Input: part model. Units: mm. Frame: model coordinates. A direction names the side the tool comes from. Give positions to 0.01 mm unless a question says otherwise; leave off trailing zeros. Write each loop counter-clockwise with the first axis right and the second up, starting at its lowest first coordinate (ties: lowest second). Pieces come first, ordered by that corner, then holes. Notation, with made-up numbers: (-36.5, 45.25) - (22.5, 45.25) arc R28 cw to (22.5, 84.25) - close; hole circle Ø1 at (24, -11.75). An arc over 180 degrees is marked (long way). Answer as a JSON object with one key per item and string values. Group by question number.
from build123d import *

# Parameters (mm, degrees)
F0_W     = 94
F0_H     = 148
F0_W_2   = 78
F0_H_2   = 136
F1_DEPTH = 2.5
F2_DEPTH = 3.2
F3_SIZE  = 3.19999
F6_DEPTH = 9
F7_R     = 5.99999
F8_R     = 2.5
F9_DEPTH = 12.1


# Not quite as in the source:
# - a fillet or chamfer is up to 0.001 mm smaller than in the source, because OpenCascade refuses the exact size


with BuildPart() as f1:
    # F0 (on Top) → F1 (new body)
    with BuildSketch(Plane.XY):
        Rectangle(F0_W, F0_H)
        with Locations((0, -2)):
            Rectangle(F0_W_2, F0_H_2, mode=Mode.SUBTRACT)
        with Locations((0, -2)):
            Rectangle(F0_W_2, F0_H_2)
    extrude(amount=-F1_DEPTH)

    # F0 (on Top) → F2 (join)
    with BuildSketch(Plane.XY):
        with Locations((0, -2)):
            Rectangle(F0_W_2, F0_H_2)
    extrude(amount=F2_DEPTH)

    # F3 (size 3.2 in the source; OpenCascade refuses exactly that, so slightly less here)
    f3_edges = [f1.edges().sort_by_distance(p)[0] for p in [
        (-39, -2, 3.2),
        (0, -70, 3.2),
        (39, -2, 3.2),
        (0, 66, 3.2),
    ]]
    chamfer(f3_edges, length=F3_SIZE)

    # F5 (on face) → F6 (join)
    with BuildSketch(Plane.XY.offset(3.2)):
        Polygon((-21.4385061716, 24.1024312943), (-19.825111455, 21.5732105668), (-14.9849273053, 13.9855483843), (-4.8680443952, 20.4391272506), (-11.3216232616, 30.5560101607), align=None)
    extrude(amount=F6_DEPTH)

    # F7 (radius 6 in the source; OpenCascade refuses exactly that, so slightly less here)
    f7_edges = [f1.edges().sort_by_distance(p)[0] for p in [
        (-9.926486, 17.212338, 12.2),
        (-16.380065, 27.329221, 12.2),
    ]]
    fillet(f7_edges, radius=F7_R)

    # F8 (on face) → F9 (cut)
    with BuildSketch(Plane(origin=(-4.3097861814, -2.749220809, 0), x_dir=(0.5377982389, -0.8430735758, 0), z_dir=(-0.8430735758, -0.5377982389, 0))):
        with Locations((-25.8497138006, 8.2)):
            Circle(F8_R)
    extrude(amount=-F9_DEPTH, mode=Mode.SUBTRACT)


solid = f1.part
1) Pin query (flat end, axial travel): P1, Ø4, axis at x = -17.5, y = 50.5, coming from the +Z side; P2, Ø6, axis at x = 16, z = 9, coming from the -Y side; P3, Ø1.5, axis at x = -28.5, z = 3, coming from the -Y side; P4, Ø4, axis at y = 27.5, z = 0.5, coming from the -X side. Return the tip coordinate at first contact, or that it passes through.
2) Cut plane C-C on z = 1.5. Return the cut outline in (x, y).
3) Line query: line 1 along Z through (x, y) = (19.5, 43.5); line 2 along Z through (x, y) = (40, 20.5); line 3 along Y through (x, z) = (-9.5, 7). Output: solid intervals per line, ascending. Write a range as from..to.
4) Reachability of faces 1 (the face through (-42, 6, 0)), 2 (the face through (-9.997, 17.167, 4.679)), 3 (the face through (-8.8, 26.6, 5.6)), 4 (the face through (-16.309, 27.374, 4.679)) from +Z, -Z, +X, -X, +Y, -Y: full face, straight path, thin tool, end or side. Return the list, or none.
5) Mould query, pull axis Z, two halves, no side actions, for faces 5 (the face through (-1, 64, 2)), 6 (the face through (-12.604, 21.253, 5.982)), 7 (the face through (-1, 1, -2.5)). Classes: +Z half, -Z half, draft (parallel to the pull), parting line (faces both ways), or undercut.
Filled in:
{
 "1": {"P1": "stops at z = 3.2", "P2": "passes through", "P3": "stops at y = -67.75", "P4": "stops at x = -47"},
 "2": {"outline": "(-37.5, -68.5) - (37.5, -68.5) - (37.5, 64.5) - (-37.5, 64.5) - close"},
 "3": {"line 1": "z = -2.5..3.2", "line 2": "z = -2.5..0", "line 3": "y = 17.55..22, 27.2..27.7"},
 "4": {"face 1": "+Z", "face 2": "+Z, +X, -Y", "face 3": "+Z, +X, +Y", "face 4": "+Z, -X, +Y"},
 "5": {"face 5": "+Z half", "face 6": "undercut", "face 7": "-Z half"}
}
